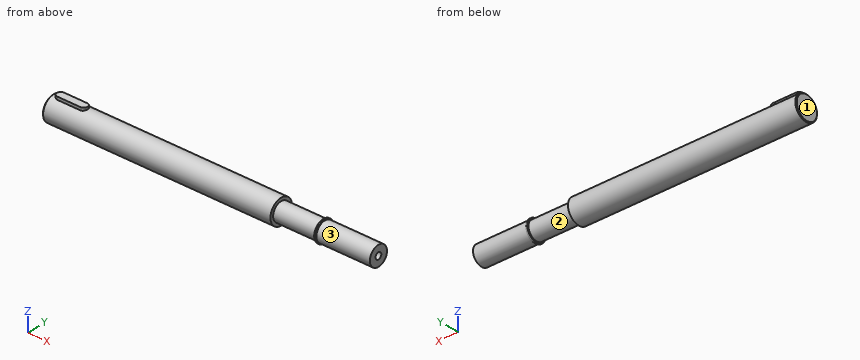
```python
from build123d import *

# Parameters (mm, degrees)
BOSS_EXTRUDE1_DEPTH        = 10
M10X1_5_TAPPED_HOLE1_D     = 8.5
M10X1_5_TAPPED_HOLE1_DEPTH = 24.5
M10X1_5_TAPPED_HOLE1_TIP   = 2.553657631


with BuildPart() as part:
    # Sketch1 → Revolve1 (revolve)
    with BuildSketch(Plane.XY, mode=Mode.PRIVATE) as revolve1_sk:
        Polygon((0, 0), (-117.829393829, 0), (-117.829393829, 15), (-116.829393829, 16), (180.170606171, 16), (180.170606171, 12), (235.320606171, 12), (235.320606171, 13.75770445), (237.320606171, 13.75770445), (237.320606171, 12.7), (307.170606171, 12.7), (307.170606171, 11), (307.170606171, 0), align=None)
    revolve(revolve1_sk.sketch.rotate(Axis((0, 0, 0), (-1, 0, 0)), 90), axis=Axis((0, 0, 0), (-1, 0, 0)))

    # Sketch2 → Boss-Extrude1 (add)
    with BuildSketch(Plane.XY.offset(19)):
        with BuildLine():
            Line((-107.829393829, 5), (-77.829393829, 5))
            ThreePointArc((-77.829393829, 5), (-72.829393829, 0), (-77.829393829, -5))
            Line((-77.829393829, -5), (-107.829393829, -5))
            ThreePointArc((-107.829393829, -5), (-112.829393829, 0), (-107.829393829, 5))
        make_face()
    extrude(amount=-BOSS_EXTRUDE1_DEPTH)

    # M10x1.5 Tapped Hole1
    with Locations(Plane(origin=(307.170606171, 0, 0), x_dir=(0, 0, -1), z_dir=(1, 0, 0))):
        with Locations((0, 0)):
            Hole(M10X1_5_TAPPED_HOLE1_D / 2, depth=M10X1_5_TAPPED_HOLE1_DEPTH)
            with Locations((0, 0, -(M10X1_5_TAPPED_HOLE1_DEPTH + M10X1_5_TAPPED_HOLE1_TIP / 2))):  # 118° drill point
                Cone(0, M10X1_5_TAPPED_HOLE1_D / 2, M10X1_5_TAPPED_HOLE1_TIP, mode=Mode.SUBTRACT)


solid = part.part
```
Work out the finished part from the listing and answer in its coordinate system (mm). Face numbers are marked on the shaded views. Round coordinates to 2 decimals unless told otherwise and drop trailing zeros. Write each loop counter-clockwise with the first axis right and the second up, starting at its lowest first coordinate (ties: lowest second). Pieces come first, ordered by that corner, then holes.
1) Consider probe 1 along X at (y, z) = (1, 12); probe 2 along Y at (x, z) = (301.25, 0); probe 3 along X at (y, z) = (-12, -9). Determine where each line is inside the solid, lowest interval first.
2) A cutting plane is placed at A-A on x = 99. Determine the outline of the cut face in (y, z).
3) Flat-ended cylindrical pins translate along their axes: P1, Ø8, axis at x = -75.5, z = -6, coming from the -Y side; P2, Ø1, axis at x = 159.5, y = -2.5, coming from the -Z side; P3, Ø6, axis at x = 258, y = -9, coming from the +Z side; P4, Ø6, axis at x = -62, z = 2, coming from the -Y side. Find the tip coordinate at first contact, or state that the pin passes through.
4) Determine the mould class of the marked faces 1, 2 and 3 for opening direction X: pulls with the +X half, pulls with the -X half, needs draft (parallel to the pull), parting line crosses it, or undercut.
5) A cutting plane is placed at B-B on x = 200. Determine the outline of the cut face in (y, z).
Entries:
1. probe 1: x = -117.83 to 180.17, 235.32 to 307.17
1. probe 2: y = -12.7 to -4.25, 4.25 to 12.7
1. probe 3: x = -117.83 to 180.17
2. outline: circle Ø32 at (0, 0)
3. P1: stops at y = -15.87
3. P2: stops at z = -15.87
3. P3: stops at z = 11.19
3. P4: stops at y = -16
4. face 1: pulls with the -X half
4. face 2: undercut
4. face 3: needs draft
5. outline: circle Ø24 at (0, 0)
